```python
from build123d import *

# Parameters (mm, degrees)
F0_R      = 38.1
F1_DEPTH  = 3.81
F1_FACE_R = 38.1
F3_R      = 26.67
F5_R      = 24.13
F6_DEPTH  = 6.35


with BuildPart() as f1:
    # F0 (on Top) → F1 (new body)
    with BuildSketch(Plane.XY):
        Circle(F0_R)
    extrude(amount=F1_DEPTH)

    # F1_face (on face) → F4 section 0
    with BuildSketch(Plane.XY.offset(3.81)):
        Circle(F1_FACE_R)
    # F3 (on offset) → F4 section 1
    with BuildSketch(Plane.XY.offset(63.5)):
        Circle(F3_R)
    loft()

    # F5 (on face) → F6 (cut)
    with BuildSketch(Plane.XY.offset(63.5)):
        Circle(F5_R)
    extrude(amount=-F6_DEPTH, mode=Mode.SUBTRACT)


solid = f1.part
```
Design review of the part built by this model. Coordinates are the model's own, in mm. A direction names the side the tool comes from. Coordinates: 2 decimals unless noted, no trailing zeros. Loops run counter-clockwise (first coordinate to the right, second up) from the corner with the lowest first, then second, coordinate; pieces in that order, holes last. Notation, with made-up numbers: (67.5, 81.25) -> (103.5, 81.25) arc R21 ccw to (103.5, 116.25) -> close; hole circle Ø5 at (-12, 11). An arc over 180 degrees is marked (long way). Answer as a JSON object with one key per item and string values.
Q1. To check wall thickness, follow L1, parallel to Z at x = 2, y = -16; L2, parallel to Y at x = 0, z = 61; L3, parallel to Y at x = 0, z = 60.5. State the ranges of each line that lie inside material, in increasing order.
Answer block:
{"L1": "z = 0 to 57.15", "L2": "y = -27.15 to -24.13, 24.13 to 27.15", "L3": "y = -27.24 to -24.13, 24.13 to 27.24"}
Q2. Tool access review of faces 1 (the cylindrical face through (23.016, 7.248, 60.369)), 2 (the cylindrical face through (-30.235, -23.183, 1.878)): name each direction out of +Z, -Z, +X, -X, +Y, -Y from which nothing blocks a thin tool from reaching the whole face with its end or side.
Answer block:
{"face 1": "+Z", "face 2": "+Z, -Z"}
Q3. Clearance check with flat-ended pins moving along their axes: pin 1 Ø1.5 at (y, z) = (-28, 21) entering from -X; pin 2 Ø12 at (y, z) = (-28.5, 45.5) entering from +X; pin 3 Ø8 at (x, z) = (23.5, 19.5) entering from -Y. State where each tip first meets the part, or that it passes through.
Answer block:
{"pin 1": "stops at x = -21.69", "pin 2": "stops at x = 20.24", "pin 3": "stops at y = -29.33"}
Q4. Take a section at B-B on z = 11.5. Give the boundary of the cut face in (x, y).
Answer block:
{"outline": "circle Ø73.25 at (0, 0)"}
Q5. The part is to be moulded in two halves that separate along X. For faces 3 (the flat face through (0, 0, 57.15)), 4 (the flat face through (-20, -14, 63.5)), 5 (the conical face through (29.6, 9.32, 40.71)), say which applies: +X half, -X half, draft (parallel to the pull), parting line (faces both ways), or undercut.
Answer block:
{"face 3": "undercut", "face 4": "draft", "face 5": "parting line"}
Q6. Take a section at C-C on z = 40.5. Give the boundary of the cut face in (x, y).
Answer block:
{"outline": "circle Ø62.15 at (0, 0)"}
Q7. Take a section at A-A on x = 0. Give the boundary of the cut face in (y, z), plus the area to 3 significant figures.
Answer block:
{"outline": "(-38.1, 0) -> (38.1, 0) -> (38.1, 3.81) -> (26.67, 63.5) -> (24.13, 63.5) -> (24.13, 57.15) -> (-24.13, 57.15) -> (-24.13, 63.5) -> (-26.67, 63.5) -> (-38.1, 3.81) -> close", "area": "3,850 mm^2"}
